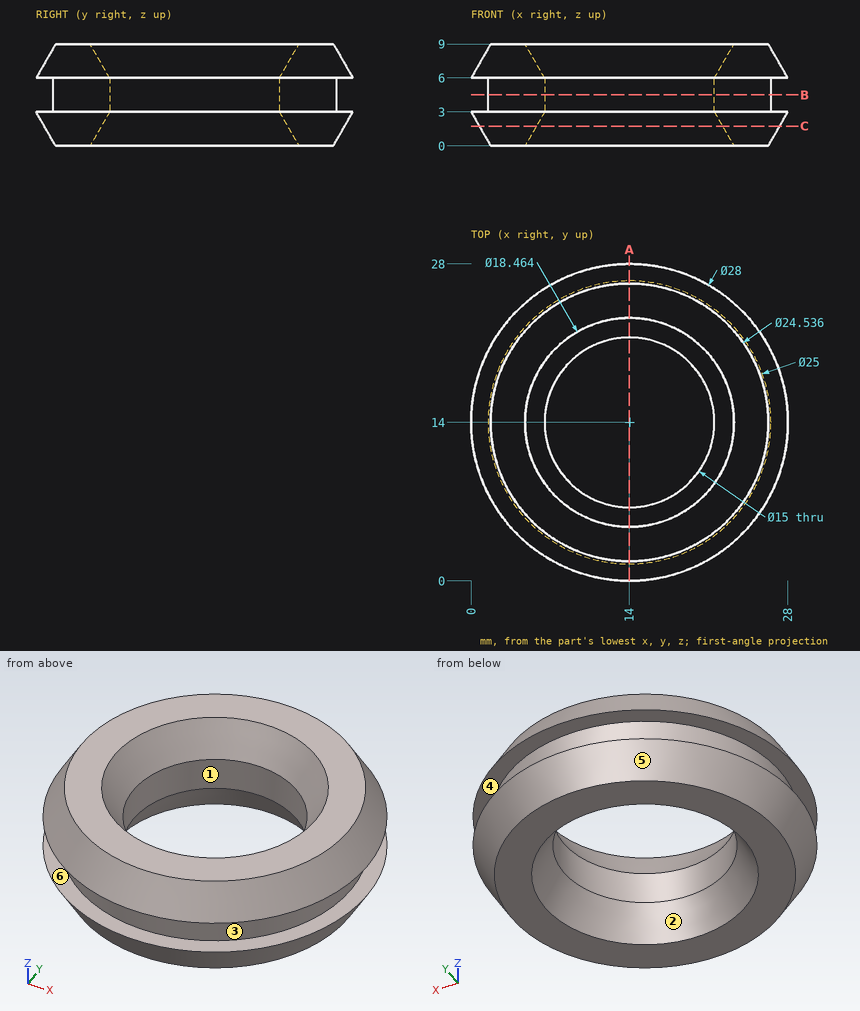
Geometry: see drawing. Coordinates: mm, zero at the bounding-box minimum. A direction names the side the tool comes from. Round coordinates to 2 decimals unless told otherwise and drop trailing zeros. Order: outer loops, then holes, each group sorted by start corner. A loop starts at its lowest first (then second) coordinate and runs counter-clockwise, first axis right, second up. Notation, with made-up numbers: (13, 34) -> (20, 34) arc R21 cw to (20, 43) -> close; hole circle Ø6 at (10.25, -29). An arc over 180 degrees is marked (long way). Answer as CSV lines item,"result".
Item 1: Section A-A, the plane x = 14. Return loops of the section in (y, z), plus the area to 3 significant figures.
A:
outline,"(0, 3) -> (1.73, 0) -> (4.77, 0) -> (6.5, 3) -> (6.5, 6) -> (4.77, 9) -> (1.73, 9) -> (0, 6) -> (1.5, 6) -> (1.5, 3) -> close; (21.5, 3) -> (23.23, 0) -> (26.27, 0) -> (28, 3) -> (26.5, 3) -> (26.5, 6) -> (28, 6) -> (26.27, 9) -> (23.23, 9) -> (21.5, 6) -> close"
area,"87.2 mm²"
Item 2: Pin query (flat end, axial travel): pin 1 Ø13.5 at (x, y) = (14, 14) entering from -Z; pin 2 Ø2 at (x, z) = (20.5, 2) entering from +Y. Return the tip coordinate at first contact, or that it passes through.
A:
pin 1,"through"
pin 2,"y = 26.57"
Item 3: Pull-direction query (X, two-part tool) for the marked faces 1, 2, 3 and 4; classes: pulls with the +X half, pulls with the -X half, needs draft (parallel to the pull), parting line crosses it, or undercut.
A:
face 1,"undercut"
face 2,"undercut"
face 3,"parting line crosses it"
face 4,"needs draft"
Item 4: Line query: L1, parallel to Y at x = 14, z = 4.45; L2, parallel to Z at x = 15.25, y = 26.5; L3, parallel to Y at x = 10.5, z = 4. Output: solid intervals per line, ascending.
A:
L1,"1.5 to 6.5, 21.5 to 26.5"
L2,"0.51 to 3, 6 to 8.49"
L3,"2 to 7.37, 20.63 to 26"
Item 5: Section B-B, the plane z = 4.5. Return loops of the section in (x, y), plus the area to 3 significant figures.
A:
outline,"circle Ø25 at (14, 14); hole circle Ø15 at (14, 14)"
area,"314 mm²"
Item 6: Reachability of the marked faces 5 and 6 from +Z, -Z, +X, -X, +Y, -Y: full face, straight path, thin tool, end or side. Return the list, or none.
A:
face 5,"-Z"
face 6,"none"
Item 7: Section C-C, the plane z = 1.75. Return loops of the section in (x, y).
A:
outline,"circle Ø26.56 at (14, 14); hole circle Ø16.44 at (14, 14)"
